```python
from build123d import *

# Parameters (mm, degrees)
BOSS_EXTRUDE1_DEPTH     = 12
CUT_EXTRUDE1_DEPTH      = 50.992671716
CUT_EXTRUDE1_DEPTH_BACK = 50.992671716
CUT_EXTRUDE2_DEPTH      = 50.992671716
CUT_EXTRUDE2_DEPTH_BACK = 50.992671716
SKETCH4_R               = 3
SKETCH4_R_2             = 1.5
SKETCH5_R               = 3
SKETCH5_R_2             = 1.5
BOSS_EXTRUDE2_DEPTH     = 2.5
FILLET1_R               = 1
FILLET2_R               = 10
SKETCH6_W               = 5
SKETCH6_H               = 10
CUT_EXTRUDE3_DEPTH      = 5
SKETCH7_W               = 5
SKETCH7_H               = 2.5
CUT_EXTRUDE4_DEPTH      = 10
SKETCH8_W               = 5
SKETCH8_H               = 10
CUT_EXTRUDE5_DEPTH      = 52.877425006


with BuildPart() as part:
    # Sketch1 → Boss-Extrude1 (new body)
    with BuildSketch(Plane.XY):
        Polygon((0, 26.132816823), (0, -47.867183177), (8, -47.867183177), (16, -10.867183177), (16, 26.132816823), align=None)
    extrude(amount=BOSS_EXTRUDE1_DEPTH)

    # Sketch3 → Cut-Extrude1 (cut, two sides: drawn at the far end of the back side and taken through both)
    with BuildSketch(Plane(origin=(8, 0, 0), x_dir=(0, 0, -1), z_dir=(1, 0, 0)).offset(-CUT_EXTRUDE1_DEPTH_BACK)):
        Polygon((-8, 26.132816823), (0, 26.132816823), (0, 18.132816823), align=None)
    extrude(amount=CUT_EXTRUDE1_DEPTH + CUT_EXTRUDE1_DEPTH_BACK, mode=Mode.SUBTRACT)

    # Sketch4 → Cut-Extrude2 (cut, two sides: drawn at the far end of the back side and taken through both)
    with BuildSketch(Plane(origin=(8, 0, 0), x_dir=(0, 0, -1), z_dir=(1, 0, 0)).offset(-CUT_EXTRUDE2_DEPTH_BACK)):
        with Locations((-6, 27.232816823)):
            Circle(SKETCH4_R)
        with Locations((-6, 27.232816823)):
            Circle(SKETCH4_R_2, mode=Mode.SUBTRACT)
    extrude(amount=CUT_EXTRUDE2_DEPTH + CUT_EXTRUDE2_DEPTH_BACK, mode=Mode.SUBTRACT)

    # Sketch5 → Boss-Extrude2 (add, symmetric)
    with BuildSketch(Plane(origin=(8, 0, 0), x_dir=(0, 0, -1), z_dir=(1, 0, 0))):
        with Locations((-6, 27.232816823)):
            Circle(SKETCH5_R)
        with Locations((-6, 27.232816823)):
            Circle(SKETCH5_R_2, mode=Mode.SUBTRACT)
    extrude(amount=BOSS_EXTRUDE2_DEPTH, both=True)

    # Fillet1
    fillet1_edges = [part.edges().sort_by_distance(p)[0] for p in [
        (8, 24.234541988, 6.101725164),
        (8, 26.132816823, 8.791057147),
    ]]
    fillet(fillet1_edges, radius=FILLET1_R)

    # Fillet2
    fillet2_edges = [part.edges().sort_by_distance(p)[0] for p in [
        (8, 18.132816823, 0),
    ]]
    fillet(fillet2_edges, radius=FILLET2_R)

    # Sketch6 → Cut-Extrude3 (cut)
    with BuildSketch(Plane(origin=(0, 0, 0), x_dir=(-1, 0, 0), z_dir=(0, 0, -1))):
        with Locations((-8, -0.867183177)):
            Rectangle(SKETCH6_W, SKETCH6_H)
        with Locations((-8, -20.867183177)):
            Rectangle(SKETCH6_W, SKETCH6_H)
    extrude(amount=-CUT_EXTRUDE3_DEPTH, mode=Mode.SUBTRACT)

    # Sketch7 → Cut-Extrude4 (cut)
    with BuildSketch(Plane.XZ.offset(15.867183177)):
        with Locations((8, 3.75)):
            Rectangle(SKETCH7_W, SKETCH7_H)
    extrude(amount=-CUT_EXTRUDE4_DEPTH, mode=Mode.SUBTRACT)

    # Sketch8 → Cut-Extrude5 (cut, through all)
    with BuildSketch(Plane(origin=(0, 0, 0), x_dir=(-1, 0, 0), z_dir=(0, 0, -1))):
        with Locations((-8, -20.867183177)):
            Rectangle(SKETCH8_W, SKETCH8_H)
    extrude(amount=-CUT_EXTRUDE5_DEPTH, mode=Mode.SUBTRACT)


solid = part.part
```
Design review of the part built by this model. Coordinates are the model's own, in mm. A direction names the side the tool comes from. Coordinates: 2 decimals unless noted, no trailing zeros. Order: outer loops, then holes, each group sorted by start corner. A loop starts at its lowest first (then second) coordinate and runs counter-clockwise, first axis right, second up. Notation, with made-up numbers: (-27.75, -24) - (28.25, -24) arc R17 ccw to (28.25, -17) - close; hole circle Ø10 at (74.5, 0). An arc over 180 degrees is marked (long way). One line per question, with ' | ' between items.
Q1. To check wall thickness, follow line 1 along Y through (x, z) = (6.7, 6); line 2 along Z through (x, y) = (9.5, -12.5); line 3 along X through (y, z) = (-8, 3). State the ranges of each line that lie inside material, in increasing order.
Answer key:
line 1: y = -47.87 to -25.87, -15.87 to 25.73, 28.73 to 30.23 | line 2: z = 0 to 2.5, 5 to 12 | line 3: x = 0 to 5.5, 10.5 to 16
Q2. The part is to be moulded in two halves that separate along Y. For faces 4 (the flat face through (8, -6, 5)), 5 (the cylindrical face through (2.712, 24.796, 7.75)), 6 (the flat face through (8, -10, 12)), say which applies: +Y half, -Y half, draft (parallel to the pull), parting line (faces both ways), or undercut.
Answer key:
face 4: undercut | face 5: +Y half | face 6: draft
Q3. For faces 1 (the flat face through (8, -5.867, 1)), 2 (the cylindrical face through (13.212, 24.796, 7.75)), 3 (the flat face through (8, -15.867, 8)), list the 3-axis set-ups (+Z, -Z, +X, -X, +Y, -Y) from which the entire face can be reached by the end or side of a thin tool; tool diameter is ignored.
Answer key:
face 1: -Z | face 2: -Z, +X, +Y | face 3: +Z, -Z
Q4. Consider section C-C, the plane y = -18.5. Give the boundary of the cut face in (x, z), then the cut area to 3 significant figures.
Answer key:
outline: (0, 0) - (5.5, 0) - (5.5, 12) - (0, 12) - close; (10.5, 0) - (14.35, 0) - (14.35, 12) - (10.5, 12) - close | area: 112 mm2
Q5. Consider section A-A, the plane y = -2. Give the boundary of the cut face in (x, z), then the cut area to 3 significant figures.
Answer key:
outline: (0, 0) - (5.5, 0) - (5.5, 5) - (10.5, 5) - (10.5, 0) - (16, 0) - (16, 12) - (0, 12) - close | area: 167 mm2
Q6. Consider section B-B, the plane x = 2.75. Give the boundary of the cut face in (y, z).
Answer key:
outline: (-47.87, 0) - (13.99, 0) arc R10 ccw to (21.06, 2.93) - (24.23, 6.1) arc R3 cw to (26.13, 8.79) - (26.13, 12) - (-47.87, 12) - close
Q7. Consider section D-D, the plane x = 14. Give the boundary of the cut face in (y, z).
Answer key:
outline: (-20.12, 0) - (13.99, 0) arc R10 ccw to (21.06, 2.93) - (24.23, 6.1) arc R3 cw to (26.13, 8.79) - (26.13, 12) - (-20.12, 12) - close
Q8. Clearance check with flat-ended pins moving along their axes: pin 1 Ø5 at (y, z) = (27.23, 6) entering from +X; pin 2 Ø2.5 at (x, z) = (5.5, 11) entering from +Y. State where each tip first meets the part, or that it passes through.
Answer key:
pin 1: stops at x = 10.5 | pin 2: stops at y = 26.16
